Build history of the part. All positions in model axes, mm. A direction names the side the tool comes from. Coordinates: 2 decimals unless noted, no trailing zeros. Use CSV: the item, a comma, the result in double quotes. Start each with the question number.
Autodesk Fusion 360 part; units mm, degrees
sketch "Esboço1" plane through (0, 0, 0) normal (0, 0, 1) x (1, 0, 0)
  circle A0 centre (-53.1, 53.1) radius 10.65
  circle A1 centre (53.1, 53.1) radius 10.65
  circle A2 centre (-53.1, -53.1) radius 10.65
  circle A3 centre (53.1, -53.1) radius 10.65
  line L0 (0, 53.1) -> (0, -53.1) construction
  line L1 (-53.1, 0) -> (53.1, 0) construction
  line L2 (-53.1, -53.1) -> (-15.5526, -15.5526) construction
  line L3 (53.1, -53.1) -> (15.5526, -15.5526) construction
  line L4 (53.1, 53.1) -> (15.5526, 15.5526) construction
  line L5 (9.5526, -15.5526) -> (-9.5526, -15.5526)
  line L6 (-15.5526, -9.5526) -> (-15.5526, 9.5526)
  line L7 (-9.5526, 15.5526) -> (9.5526, 15.5526)
  line L8 (15.5526, 9.5526) -> (15.5526, -9.5526)
  line L9 (15.5526, -15.5526) -> (-15.5526, 15.5526) construction
  line L10 (-15.5526, -15.5526) -> (15.5526, 15.5526) construction
  line L11 (-42.45, 53.1) -> (-4.9431, 15.5526) construction
  line L12 (-53.1, 42.45) -> (-15.5526, 4.9026) construction
  line L13 (-23.6965, 34.3263) -> (-29.0114, 29.0114) construction
  line L14 (-34.3263, 23.6763) -> (-29.0114, 29.0114) construction
  spline S0 degree 2 poles (-42.45, 53.1) (-26.354, 31.6689) (-4.9431, 15.5526) knots 0 0 0 5.336996 5.336996 5.336996 weights 1 3 1
  spline S1 degree 2 poles (-53.1, 42.45) (-31.6689, 26.3439) (-15.5526, 4.9026) knots 0 0 0 5.339953 5.339953 5.339953 weights 1 3 1
  arc A4 (-9.5526, 15.5526) -> (-15.5526, 9.5526) centre (-9.5526, 9.5526) ccw
  spline S2 degree 2 poles (42.45, 53.1) (26.354, 31.6689) (4.9431, 15.5526) knots 0 0 0 5.336996 5.336996 5.336996 weights 1 3 1
  spline S3 degree 2 poles (53.1, 42.45) (31.6689, 26.3439) (15.5526, 4.9026) knots 0 0 0 5.339953 5.339953 5.339953 weights 1 3 1
  spline S4 degree 2 poles (-53.1, -42.45) (-31.6689, -26.3439) (-15.5526, -4.9026) knots 0 0 0 5.339953 5.339953 5.339953 weights 1 3 1
  spline S5 degree 2 poles (-42.45, -53.1) (-26.354, -31.6689) (-4.9431, -15.5526) knots 0 0 0 5.336996 5.336996 5.336996 weights 1 3 1
  spline S6 degree 2 poles (42.45, -53.1) (26.354, -31.6689) (4.9431, -15.5526) knots 0 0 0 5.336996 5.336996 5.336996 weights 1 3 1
  spline S7 degree 2 poles (53.1, -42.45) (31.6689, -26.3439) (15.5526, -4.9026) knots 0 0 0 5.339953 5.339953 5.339953 weights 1 3 1
  arc A5 (15.5526, 9.5526) -> (9.5526, 15.5526) centre (9.5526, 9.5526) ccw
  arc A6 (-15.5526, -9.5526) -> (-9.5526, -15.5526) centre (-9.5526, -9.5526) ccw
  arc A7 (9.5526, -15.5526) -> (15.5526, -9.5526) centre (9.5526, -9.5526) ccw
  dimension "d1" = 106.2
  dimension "d2" = 106.2
  dimension "d3" = 21.3
  dimension "d4" = 21.3
  dimension "d5" = 21.3
  dimension "d6" = 21.3
  dimension "d12" = 6
  dimension "d13" = 106.2
  dimension "d20" = 6
  dimension "d21" = 6
  dimension "d22" = 6
extrude "Extrusão1" add sketch "Esboço1" along normal blind 5
1. Flat gauge pins, fed straight in: pin 1 (1 mm diameter, centred on y = -40, z = 3.5, fed in from +X); pin 2 (2 mm diameter, centred on y = -35, z = 1, fed in from +X); pin 3 (1.5 mm diameter, centred on x = -17, z = 3.5, fed in from +Y). Where does each tip first touch, or does it go through?
2. Pull direction X, two halves, no side cores. Call faces 4 (the flat face through (0, -4, 5)), 5 (the cylindrical face through (60.875, -60.378, 2.465)), 6 (the flat face through (0, -15.553, 2)), 7 (the flat face through (15.553, 0, 2)): pulls with the +X half, pulls with the -X half, needs draft (parallel to the pull), parting line crosses it, or undercut.
3. Drill centre lines: line 1 along Y through (x, z) = (-28, 3.7); line 2 along Y through (x, z) = (-50, 1); line 3 along X through (y, z) = (37, 0.7). Where is each one in solid material? Low to high. Write a range as from..to.
4. 3-axis set-ups, long thin cutter, end or side, ignore diameter. For faces 1 (the flat face through (0, 15.553, 2)), 2 (the cylindrical face through (-60.378, -60.875, 2.465)), 3 (the flat face through (-15.553, 0, 2)): which of +Z, -Z, +X, -X, +Y, -Y reach the whole face in a straight line?
Established:
1,pin 1,"stops at x = 50.51"
1,pin 2,"stops at x = 44.6"
1,pin 3,"stops at y = 25.39"
2,face 4,"needs draft"
2,face 5,"undercut"
2,face 6,"undercut"
2,face 7,"pulls with the +X half"
3,line 1,"y = -34.77..-20.92, 20.92..34.77"
3,line 2,"y = -63.29..-40.11, 40.11..63.29"
3,line 3,"x = -45.9..-29.94, 29.94..45.9"
4,face 1,"+Z, -Z, +Y"
4,face 2,"+Z, -Z"
4,face 3,"+Z, -Z, -X"
